Autodesk Fusion 360 part; units mm, degrees
sketch "Sketch1" plane through (0, 0, 0) normal (0, 1, 0) x (1, 0, 0)
  circle A0 centre (0, 0) radius 17.095
  circle A1 centre (0, 0) radius 32.5
  line L0 (-21.05, 10) -> (-28.55, 10)
  line L1 (-28.55, 10) -> (-28.55, -10)
  line L2 (-28.55, -10) -> (-21.05, -10)
  line L3 (-21.05, -10) -> (-21.05, 10)
  line L4 (-21.05, 0) -> (0, 0)
  line L5 (0, 0) -> (-19.4454, 19.4454)
  circle A2 centre (-19.4454, 19.4454) radius 0.5
  line L6 (-10, -21.05) -> (-10, -28.55)
  line L7 (10, -28.55) -> (10, -21.05)
  line L8 (-10, -28.55) -> (10, -28.55)
  line L9 (10, -21.05) -> (-10, -21.05)
  circle A3 centre (-19.4454, -19.4454) radius 0.5
  line L10 (21.05, -10) -> (28.55, -10)
  line L11 (28.55, 10) -> (21.05, 10)
  line L12 (28.55, -10) -> (28.55, 10)
  line L13 (21.05, 10) -> (21.05, -10)
  circle A4 centre (19.4454, -19.4454) radius 0.5
  line L14 (10, 21.05) -> (10, 28.55)
  line L15 (-10, 28.55) -> (-10, 21.05)
  line L16 (10, 28.55) -> (-10, 28.55)
  line L17 (-10, 21.05) -> (10, 21.05)
  circle A5 centre (19.4454, 19.4454) radius 0.5
  line L18 (17.3241, -8.1317) -> (8.1317, -17.3241)
  line L19 (0, 0) -> (12.7279, -12.7279)
  line L20 (10.253, -19.4454) -> (8.1317, -17.3241)
  line L21 (8.1317, -17.3241) -> (11.3137, -14.1421)
  line L22 (11.3137, -14.1421) -> (13.435, -16.2635)
  line L23 (13.435, -16.2635) -> (10.253, -19.4454)
  line L24 (19.4454, -10.253) -> (17.3241, -8.1317)
  line L25 (17.3241, -8.1317) -> (14.1421, -11.3137)
  line L26 (14.1421, -11.3137) -> (16.2635, -13.435)
  line L27 (16.2635, -13.435) -> (19.4454, -10.253)
  line L28 (11.844, -17.8544) -> (13.6118, -19.6222)
  circle A6 centre (13.6118, -19.6222) radius 0.5
  line L29 (17.8544, -11.844) -> (19.6222, -13.6118)
  circle A7 centre (19.6222, -13.6118) radius 0.5
  circle A8 centre (-13.6118, 19.6222) radius 0.5
  circle A9 centre (-19.6222, 13.6118) radius 0.5
  point P0 (0, -21.05)
  point P1 (21.05, 0)
  point P2 (0, 21.05)
  dimension "d1" = 34.19
  dimension "d2" = 65
  dimension "d4" = 21.05
  dimension "d5" = 20
  dimension "d6" = 7.5
  dimension "d7" = 27.5
  dimension "d8" = 1
  dimension "d9" = 45
  dimension "d11" = 360
  dimension "d13" = 13
  dimension "d14" = 18
  dimension "d15" = 3
  dimension "d16" = 4.5
  dimension "d17" = 3
  dimension "d18" = 4.5
  dimension "d19" = 2.5
  dimension "d20" = 1
  dimension "d21" = 2.5
  dimension "d22" = 1
  dimension "d24" = 360
extrude "Extrude1" add sketch "Sketch1" along normal blind 12.45 contours L0 L1 L2 L3 | L6 L7 L8 L9 | L10 L11 L12 L13 | L14 L15 L16 L17 makes body 1 at (3.3333, 4.15, 21.05) makes body 2 at (21.05, 4.15, -3.3333) makes body 3 at (-21.05, 4.15, 3.3333) makes body 4 at (-3.3333, 4.15, -21.05)
extrude "Extrude2" add sketch "Sketch1" along normal blind 2 contours L18 L24 L25 L26 L27 | L18 L20 L21 L22 L23 | A1 bodies 1 2 3 4
extrude "Extrude3" add 4 faces at (-26.05, 12.45, 3.3333) (-3.3333, 12.45, 23.55) (23.55, 12.45, -3.3333) (3.3333, 12.45, -23.55) along direction (0, 1, 0) blind 1.8 on bodies 1 bodies 1
sketch "Sketch2" plane through (0, 0, 28.55) normal (0, 0, 1) x (1, 0, 0)
  line L0 (-10, 2) -> (10, 2)
  line L1 (10, 2) -> (10, 14.25)
  line L2 (10, 14.25) -> (-10, 14.25)
  line L3 (-10, 14.25) -> (-10, 2)
  circle A0 centre (0, 12.245) radius 1
  dimension "d31" = 2
  dimension "d32" = 12.245
extrude "Extrude4" add 4 faces at (-3.3333, 14.25, 23.55) (23.55, 14.25, -3.3333) (3.3333, 14.25, -23.55) (-26.05, 14.25, 3.3333) along direction (0, 1, 0) blind 3 on bodies 1 bodies 1
sketch "Sketch3" plane through (28.55, 0, 0) normal (1, 0, 0) x (0, 0, -1)
  line L0 (-10, 2) -> (10, 2)
  line L1 (10, 2) -> (10, 17.25)
  line L2 (10, 17.25) -> (-10, 17.25)
  line L3 (-10, 17.25) -> (-10, 2)
  circle A0 centre (0, 12.445) radius 1
  dimension "d35" = 2
  dimension "d36" = 12.445
extrude "Extrude5" cut sketch "Sketch3" against normal blind 60 contours A0 bodies 1
extrude "Extrude6" cut sketch "Sketch2" against normal blind 60 contours A0 bodies 1
Could you check a few things on this model? Use its own coordinates, in mm. A direction names the side the tool comes from. Round coordinates to 2 decimals unless told otherwise and drop trailing zeros. Write each loop counter-clockwise with the first axis right and the second up, starting at its lowest first coordinate (ties: lowest second). Pieces come first, ordered by that corner, then holes. Notation, with made-up numbers: (-27.75, 18) -> (6.25, 18) arc R21 ccw to (6.25, 48) -> close; hole circle Ø3 at (-14, 42.5). An arc over 180 degrees is marked (long way). Use a Markdown table: item, result.
1. For pin 1 Ø4 at (x, y) = (24, 6.5) entering from +Z; pin 2 Ø1.5 at (y, z) = (11, 9) entering from -X; pin 3 Ø2 at (x, y) = (-4, 13) entering from +Z; pin 4 Ø1.5 at (y, z) = (9.5, -19.5) entering from +X, each with a flat end and sliding along its axis, tell me the tip position at first contact or that it passes through.
Answer key:
| item | result |
|---|---|
| pin 1 | stops at z = 10 |
| pin 2 | stops at x = -28.55 |
| pin 3 | stops at z = 28.55 |
| pin 4 | passes through |
2. If we section it at B-B (x = 0): List the corners of the cut face in (y, z) for me (3 decimals), then the cut area to 3 significant figures.
Answer key:
| item | result |
|---|---|
| outline | (0, -32.5) -> (2, -32.5) -> (2, -28.55) -> (11.245, -28.55) -> (11.245, -21.05) -> (2, -21.05) -> (2, -17.095) -> (0, -17.095) -> close; (0, 17.095) -> (2, 17.095) -> (2, 21.05) -> (11.245, 21.05) -> (11.245, 28.55) -> (2, 28.55) -> (2, 32.5) -> (0, 32.5) -> close; (13.245, -28.55) -> (17.25, -28.55) -> (17.25, -21.05) -> (13.245, -21.05) -> close; (13.245, 21.05) -> (17.25, 21.05) -> (17.25, 28.55) -> (13.245, 28.55) -> close |
| area | 260 mm^2 |
3. If we section it at A-A (z = 0): List the corners of the cut face in (x, y) for me (3 decimals), then the cut area to 3 significant figures.
Answer key:
| item | result |
|---|---|
| outline | (-32.5, 0) -> (-17.095, 0) -> (-17.095, 2) -> (-21.05, 2) -> (-21.05, 11.445) -> (-28.55, 11.445) -> (-28.55, 2) -> (-32.5, 2) -> close; (-28.55, 13.445) -> (-21.05, 13.445) -> (-21.05, 17.25) -> (-28.55, 17.25) -> close; (17.095, 0) -> (32.5, 0) -> (32.5, 2) -> (28.55, 2) -> (28.55, 11.445) -> (21.05, 11.445) -> (21.05, 2) -> (17.095, 2) -> close; (21.05, 13.445) -> (28.55, 13.445) -> (28.55, 17.25) -> (21.05, 17.25) -> close |
| area | 260 mm^2 |
4. Please list where these lines run through material, in increasing order: probe 1 along X at (y, z) = (14, 6); probe 2 along Y at (x, z) = (0, 26) (3 decimals).
Answer key:
| item | result |
|---|---|
| probe 1 | x = -28.55 to -21.05, 21.05 to 28.55 |
| probe 2 | y = 0 to 11.245, 13.245 to 17.25 |
5. If we section it at D-D (x = 11): List the corners of the cut face in (y, z) for me, then the cut area to 3 significant figures.
Answer key:
| item | result |
|---|---|
| outline | (0, -30.58) -> (2, -30.58) -> (2, -13.09) -> (0, -13.09) -> close; (0, 13.09) -> (2, 13.09) -> (2, 30.58) -> (0, 30.58) -> close |
| area | 70.0 mm^2 |
6. We'd pull the mould along Z, two halves only. Please class faces 6 (the face through (24.85, 11.47, 0.22)), 7 (the face through (25, 10, 10)), 8 (the face through (-10, 10, -25)), 9 (the face through (0, 10, -28.55)): +Z half, -Z half, draft (parallel to the pull), parting line (faces both ways), or undercut.
Answer key:
| item | result |
|---|---|
| face 6 | undercut |
| face 7 | +Z half |
| face 8 | draft |
| face 9 | -Z half |
7. If we section it at C-C (y = 6.75): List the corners of the cut face in (x, z) for me.
Answer key:
| item | result |
|---|---|
| outline | (-28.55, -10) -> (-21.05, -10) -> (-21.05, 10) -> (-28.55, 10) -> close; (-10, -28.55) -> (10, -28.55) -> (10, -21.05) -> (-10, -21.05) -> close; (-10, 21.05) -> (10, 21.05) -> (10, 28.55) -> (-10, 28.55) -> close; (21.05, -10) -> (28.55, -10) -> (28.55, 10) -> (21.05, 10) -> close |
8. Which directions (+Z, -Z, +X, -X, +Y, -Y) give clear straight access to the entire face, cutting with the end or side of a thin tool? Please do faces 1 (the face through (-21.05, 10, 0)), 2 (the face through (28.55, 10, 0)), 3 (the face through (25, 10, -10)), 4 (the face through (0, 10, 21.05)), 5 (the face through (-25, 10, 10)).
Answer key:
| item | result |
|---|---|
| face 1 | +Z, -Z, +Y |
| face 2 | +Z, -Z, +X, +Y |
| face 3 | -Z, +X, -X, +Y |
| face 4 | +X, -X, +Y |
| face 5 | +Z, +X, -X, +Y |
